Autodesk Fusion 360 part; units mm, degrees
sketch "Base" plane through (0, 0, 0) normal (0, 0, 1) x (1, 0, 0)
  line L0 (-9.4551, 20.4231) -> (10.5449, 20.4231)
  line L1 (20.2949, 5.4231) -> (20.2949, -19.5769)
  line L2 (20.2949, -19.5769) -> (-20.2051, -19.5769)
  line L3 (-20.2051, -19.5769) -> (-20.2051, 5.4231)
  line L4 (-20.2051, 5.4231) -> (-9.4551, 5.4231)
  line L5 (-9.4551, 5.4231) -> (-9.4551, 20.4231)
  line L6 (10.5449, 20.4231) -> (10.5449, 5.4231)
  line L7 (10.5449, 5.4231) -> (20.2949, 5.4231)
  dimension "d1" = 40
  dimension "d2" = 40.5
  dimension "d3" = 25
  dimension "d4" = 25
  dimension "d5" = 10.75
  dimension "d6" = 20
extrude "Extrude1" add sketch "Base" along normal blind 3
sketch "Messurements" plane through (0, 0, 3) normal (0, 0, 1) x (-1, 0, 0)
  line L0 (-10.5449, -5.4231) -> (-10.5449, -20.4231)
  line L1 (-10.5449, -20.4231) -> (9.4551, -20.4231)
  line L2 (9.4551, -20.4231) -> (9.4551, -5.4231)
  line L3 (9.4551, -5.4231) -> (20.2051, -5.4231)
  line L4 (20.2051, -5.4231) -> (20.2051, 19.5769)
  line L5 (20.2051, 19.5769) -> (-20.2949, 19.5769)
  line L6 (-20.2949, 19.5769) -> (-20.2949, -5.4231)
  line L7 (-20.2949, -5.4231) -> (-10.5449, -5.4231)
  line L8 (20.2051, 14.0769) -> (-20.2949, 14.0769)
  line L9 (9.4551, -5.4231) -> (-10.5449, -5.4231)
  line L10 (9.4551, -8.4231) -> (-10.5449, -8.4231)
  circle A0 centre (-5.2949, 4.5769) radius 2.5
  circle A1 centre (9.6801, 4.5769) radius 3.125
  dimension "d9" = 5.5
  dimension "d10" = 3
  dimension "d11" = 5
  dimension "d12" = 6.25
  dimension "d13" = 15
  dimension "d14" = 10
  dimension "d15" = 10
  dimension "d16" = 10.525
extrude "Extrude2" cut sketch "Messurements" against normal blind 2 contours A0
extrude "Extrude3" add sketch "Messurements" along normal blind 8 contours A1
extrude "Extrude4" add sketch "Messurements" along normal blind 5 contours L4 L5 L6 L8
extrude "Extrude5" add sketch "Messurements" along normal blind 13 contours L0 L2 L9 L10
sketch "Other" plane through (0, 0, 8) normal (0, 0, 1) x (-1, 0, 0)
  line L0 (20.2051, 19.5769) -> (-20.2949, 19.5769)
  line L1 (-20.2949, 19.5769) -> (-20.2949, 14.0769)
  line L2 (-20.2949, 14.0769) -> (20.2051, 14.0769)
  line L3 (20.2051, 14.0769) -> (20.2051, 19.5769)
  line L4 (20.2051, 14.0769) -> (-20.2949, 14.0769)
  line L5 (-20.2949, 16.5769) -> (20.2051, 16.5769)
  dimension "d28" = 2.5
extrude "Extrude6" add sketch "Other" along normal blind 8 contours L0 L1 L3 L5
sketch "Attachment2" plane through (0, -16.5769, 0) normal (0, 1, 0) x (-1, 0, 0)
  line L0 (-20.2949, 8) -> (20.2051, 8)
  line L1 (20.2051, 8) -> (20.2051, 16)
  line L2 (20.2051, 16) -> (-20.2949, 16)
  line L3 (-20.2949, 16) -> (-20.2949, 8)
  circle A0 centre (-14.9949, 12.3) radius 1.3
  circle A1 centre (14.5051, 12.3) radius 1.3
  dimension "d31" = 2.6
  dimension "d32" = 3.7
  dimension "d33" = 5.3
  dimension "d34" = 2.6
  dimension "d35" = 5.7
  dimension "d36" = 3.7
extrude "Extrude7" cut sketch "Attachment2" against normal through all contours A0
extrude "Extrude8" cut sketch "Attachment2" against normal through all contours A1
sketch "Attachment" plane through (0, 8.4231, 0) normal (0, 1, 0) x (-1, 0, 0)
  line L0 (-10.5449, 3) -> (9.4551, 3)
  line L1 (9.4551, 3) -> (9.4551, 16)
  line L2 (9.4551, 16) -> (-10.5449, 16)
  line L3 (-10.5449, 16) -> (-10.5449, 3)
  circle A0 centre (-0.9949, 12.3) radius 1.3
  dimension "d39" = 2.6
  dimension "d40" = 3.7
  dimension "d41" = 9.55
extrude "Extrude9" cut sketch "Attachment" against normal blind 4 contours A0
Work out the finished part from the listing and answer in its coordinate system (mm). A direction names the side the tool comes from. Coordinates: 2 decimals unless noted, no trailing zeros. Write each loop counter-clockwise with the first axis right and the second up, starting at its lowest first coordinate (ties: lowest second). Pieces come first, ordered by that corner, then holes. Notation, with made-up numbers: M 46.5,76 L 84.5,76 A7 ccw 84.5,84 Z; hole C -34.5,75 d2. An arc over 180 degrees is marked long. Answer as CSV lines item,"result". Start each with the question number.
Item 1: Section B-B on x = -5 is taken. Write down the section's boundary in (y, z), and give its area (4 significant figures).
Item 2: Section D-D on y = 17 is taken. Write down the section's boundary in (x, z), and give its area (3 significant figures).
Item 3: Consider L1, parallel to Y at x = 1, z = 9; L2, parallel to Y at x = -9, z = 4.5; L3, parallel to X at y = 8, z = 10.5. Determine where each line is inside the solid, lowest interval first.
Item 4: Section C-C on z = 4 is taken. Write down the section's boundary in (x, y) (3 decimals).
Item 5: A tool of negligible diameter and unlimited length cuts with its end or side. For faces 1 (the face through (5, -5, 1)), 2 (the face through (-15, 5.423, 1)), 3 (the face through (0, -16.577, 12)), from which of +Z, -Z, +X, -X, +Y, -Y can it reach the whole face along a straight path? Write none if from no direction.
Item 6: Section A-A on z = 12.3 is taken. Write down the section's boundary in (x, y), and give its area (3 significant figures).
Item 7: Determine the mould class of faces 4 (the face through (1.16, 6.94, 13.59)), 5 (the face through (-15.745, -18.056, 12.69)), 6 (the face through (0, -4, 0)), 7 (the face through (0, -15, 8)) for opening direction Z: released by +Z, released by -Z, zero draft, split by the parting line, or undercut.
Item 8: Flat-ended cylindrical pins translate along their axes: P1, Ø1.5, axis at x = 5, y = -3.5, coming from the +Z side; P2, Ø3.5, axis at x = 13.5, z = 1, coming from the +Y side; P3, Ø3, axis at x = -15, z = 10, coming from the +Y side. Find the tip coordinate at first contact, or state that the pin passes through.
Checks:
1,outline,"M -19.58,0 L 20.42,0 L 20.42,3 L 8.42,3 L 8.42,16 L 5.42,16 L 5.42,3 L -14.08,3 L -14.08,8 L -16.58,8 L -16.58,16 L -19.58,16 Z"
1,area,"210.5 mm²"
2,outline,"M -9.46,0 L 10.54,0 L 10.54,3 L -9.46,3 Z"
2,area,"60.0 mm²"
3,L1,"y = -19.58 to -16.58, 5.42 to 8.42"
3,L2,"y = -19.58 to -14.08, -7.63 to -1.53, 5.42 to 8.42"
3,L3,"x = -9.46 to 10.54"
4,outline,"M -20.205,-19.577 L 20.295,-19.577 L 20.295,-14.077 L -20.205,-14.077 Z; C -9.68,-4.577 d6.25; M -9.455,5.423 L 10.545,5.423 L 10.545,8.423 L -9.455,8.423 Z"
5,face 1,"+Z"
5,face 2,"+Z, -Z, -X, +Y"
5,face 3,"+Z, +X, -X"
6,outline,"M -20.21,-19.58 L -15.81,-19.58 L -15.81,-16.58 L -20.21,-16.58 Z; M -13.21,-19.58 L 13.69,-19.58 L 13.69,-16.58 L -13.21,-16.58 Z; M -9.46,5.42 L -0.31,5.42 L -0.31,8.42 L -9.46,8.42 Z; M 2.29,5.42 L 10.54,5.42 L 10.54,8.42 L 2.29,8.42 Z; M 16.29,-19.58 L 20.29,-19.58 L 20.29,-16.58 L 16.29,-16.58 Z"
6,area,"158 mm²"
7,face 4,"undercut"
7,face 5,"undercut"
7,face 6,"released by -Z"
7,face 7,"released by +Z"
8,P1,"stops at z = 1"
8,P2,"stops at y = 5.42"
8,P3,"stops at y = -16.58"
